Design review of the part shown in the three views and the two pictorial views. Dimensions are in mm from the part's minimum x, y and z. Give positions to 0.01 mm unless a question says otherwise; leave off trailing zeros. Write each loop counter-clockwise with the first axis right and the second up, starting at its lowest first coordinate (ties: lowest second). Pieces come first, ordered by that corner, then holes. Notation, with made-up numbers: M 56,-13.5 L 104,-13.5 A26 cw 104,10.5 Z; hole C -26,79.25 d6. An arc over 180 degrees is marked long. Write item = value, one per line.
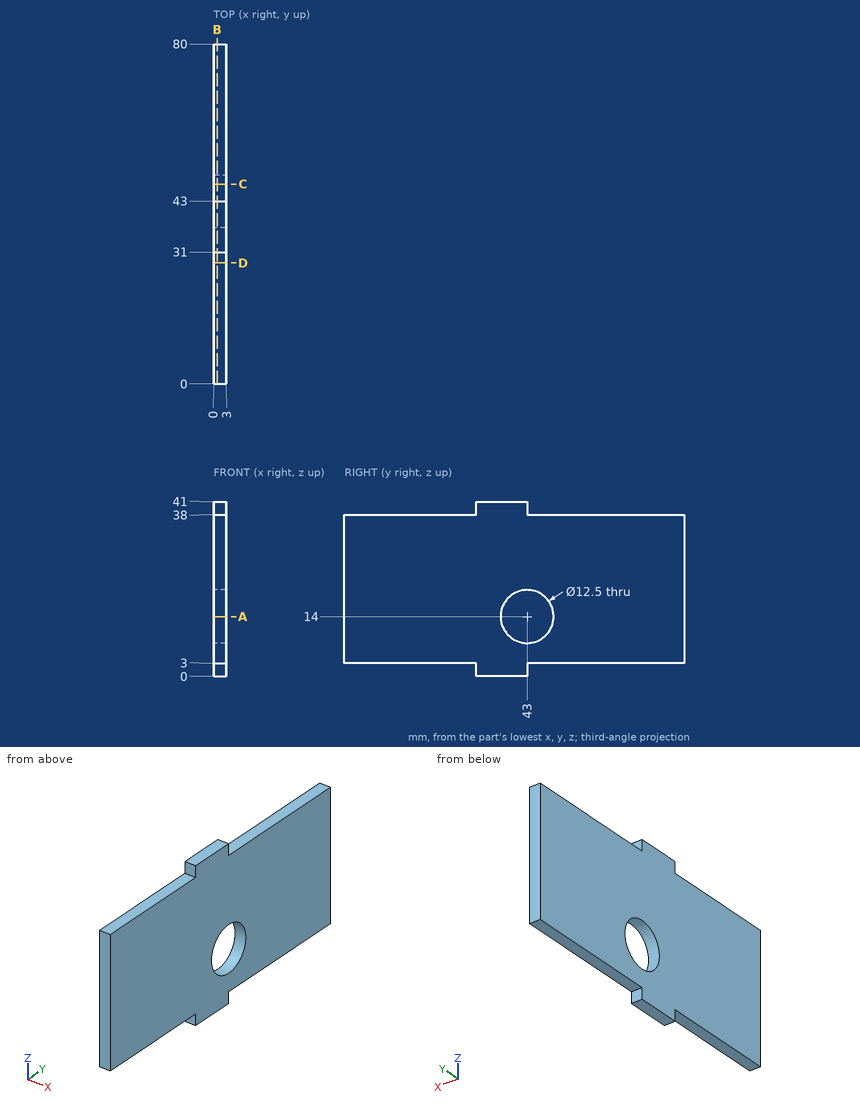
1. We need section B-B, the plane x = 0.8. Write out the cut boundary in (y, z), then the cut area to 3 significant figures.
Responses:
outline = M 0,3 L 31,3 L 31,0 L 43,0 L 43,3 L 80,3 L 80,38 L 43,38 L 43,41 L 31,41 L 31,38 L 0,38 Z; hole C 43,14 d12.5
area = 2,750 mm2
2. We need section C-C, the plane y = 47. Write out the cut boundary in (x, z).
Responses:
outline = M 0,3 L 3,3 L 3,9.2 L 0,9.2 Z; M 0,18.8 L 3,18.8 L 3,38 L 0,38 Z
3. We need section D-D, the plane y = 28.5. Write out the cut boundary in (x, z).
Responses:
outline = M 0,3 L 3,3 L 3,38 L 0,38 Z
4. Insertion check: P1, Ø1.5, axis at x = 1.5, y = 15.5, coming from the +Z side; P2, Ø0.9, axis at x = 1, y = 15, coming from the -Z side; P3, Ø1.5, axis at x = 2, z = 39, coming from the +Y side. Each pin has a flat end and moves straight along its axis. Give the tip position at first contact, or say it passes through.
Responses:
P1 = 38
P2 = 3
P3 = 43
5. We need section A-A, the plane z = 14. Write out the cut boundary in (x, y).
Responses:
outline = M 0,0 L 3,0 L 3,36.75 L 0,36.75 Z; M 0,49.25 L 3,49.25 L 3,80 L 0,80 Z
6. For line 1 along Z through (x, y) = (0.7, 23); line 2 along Z through (x, y) = (1.1, 48.5); line 3 along Z through (x, y) = (2.65, 40.5), list the stretches that pass through material, from the lowest coordinate up. Write a range as from..to.
Responses:
line_1 = 3..38
line_2 = 3..11.03, 16.97..38
line_3 = 0..8.27, 19.73..41
